Input: part model. Units: mm. Frame: model coordinates. Face numbers are marked on the shaded views. A direction names the side the tool comes from. Coordinates: 2 decimals unless noted, no trailing zeros. Order: outer loops, then holes, each group sorted by start corner. A loop starts at its lowest first (then second) coordinate and runs counter-clockwise, first axis right, second up. Notation, with made-up numbers: (52, 30.5) -> (103, 30.5) arc R36 ccw to (103, 68.5) -> close; hole circle Ø2 at (5, -25). An arc over 180 degrees is marked (long way). Write each question's results on one line, items separated by ' | '.
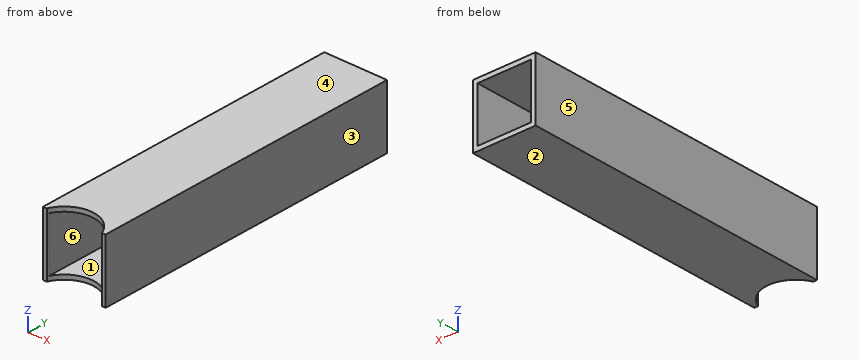
```python
from build123d import *

# Parameters (mm, degrees)
SKETCH1_W                = 44.45
SKETCH1_H                = 44.45
SKETCH1_W_2              = 38.1
SKETCH1_H_2              = 38.1
BOSS_EXTRUDE1_DEPTH      = 95.25
BOSS_EXTRUDE1_DEPTH_BACK = 95.25
SKETCH2_W                = 44.45
SKETCH2_H                = 44.45
SKETCH2_W_2              = 38.1
SKETCH2_H_2              = 38.1
BOSS_EXTRUDE2_DEPTH      = 31.75
SKETCH3_R                = 21.082
CUT_EXTRUDE1_DEPTH       = 45.45


with BuildPart() as part:
    # Sketch1 → Boss-Extrude1 (new body, two sides)
    with BuildSketch(Plane(origin=(0, 0, 0), x_dir=(1, 0, 0), z_dir=(0, 1, 0))) as boss_extrude1_sk:
        Rectangle(SKETCH1_W, SKETCH1_H)
        Rectangle(SKETCH1_W_2, SKETCH1_H_2, mode=Mode.SUBTRACT)
    extrude(amount=BOSS_EXTRUDE1_DEPTH)
    extrude(boss_extrude1_sk.sketch, amount=-BOSS_EXTRUDE1_DEPTH_BACK)

    # Sketch2 → Boss-Extrude2 (add)
    with BuildSketch(Plane.XZ.offset(95.25)):
        Rectangle(SKETCH2_W, SKETCH2_H)
        Rectangle(SKETCH2_W_2, SKETCH2_H_2, mode=Mode.SUBTRACT)
    extrude(amount=BOSS_EXTRUDE2_DEPTH)

    # Sketch3 → Cut-Extrude1 (cut, through all)
    with BuildSketch(Plane.XY.offset(22.225)):
        with Locations((0, -134.9375)):
            Circle(SKETCH3_R)
    extrude(amount=-CUT_EXTRUDE1_DEPTH, mode=Mode.SUBTRACT)


solid = part.part
```
(1) Cut plane D-D, the plane x = -9. Return loops of the section in (y, z) (3 decimals).
Return value:
outline: (-115.873, -22.225) -> (95.25, -22.225) -> (95.25, -19.05) -> (-115.873, -19.05) -> close; (-115.873, 19.05) -> (95.25, 19.05) -> (95.25, 22.225) -> (-115.873, 22.225) -> close
(2) Cut plane A-A, the plane y = -49. Return loops of the section in (x, z) (3 decimals), plus the area to 3 significant figures.
Return value:
outline: (-22.225, -22.225) -> (22.225, -22.225) -> (22.225, 22.225) -> (-22.225, 22.225) -> close; hole (-19.05, -19.05) -> (19.05, -19.05) -> (19.05, 19.05) -> (-19.05, 19.05) -> close | area: 524 mm2
(3) Line query: line 1 along Z through (x, y) = (-0.5, -103.5) (3 decimals). Output: solid intervals per line, ascending. Write a range as from..to.
Return value:
line 1: -22.225..-19.05, 19.05..22.225
(4) Cut plane C-C, the plane x = 5.5. Return loops of the section in (y, z) (3 decimals).
Return value:
outline: (-114.586, -22.225) -> (95.25, -22.225) -> (95.25, -19.05) -> (-114.586, -19.05) -> close; (-114.586, 19.05) -> (95.25, 19.05) -> (95.25, 22.225) -> (-114.586, 22.225) -> close
(5) Reachability of the marked faces 5 and 6 from +Z, -Z, +X, -X, +Y, -Y: full face, straight path, thin tool, end or side. Return the list, or none.
Return value:
face 5: +Z, -Z, -X, +Y, -Y | face 6: +Y, -Y
(6) Mould query, pull axis Z, two halves, no side actions, for the marked faces 1, 2, 3 and 4. Classes: +Z half, -Z half, draft (parallel to the pull), parting line (faces both ways), or undercut.
Return value:
face 1: undercut | face 2: -Z half | face 3: draft | face 4: +Z half
(7) Pin query (flat end, axial travel): P1, Ø8, axis at x = 5.5, z = 17, coming from the -Y side. Return the tip coordinate at first contact, or that it passes through.
Return value:
P1: y = -115.84
